The drawing under review shows one solid part. Ordinate dimensions are in mm from its lowest x, y, z. A direction names the side the tool comes from. Give positions to 0.01 mm unless a question says otherwise; leave off trailing zeros. Write each loop counter-clockwise with the first axis right and the second up, starting at its lowest first coordinate (ties: lowest second). Pieces come first, ordered by that corner, then holes. Notation, with made-up numbers: (58, -16) -> (86, -16) arc R26 ccw to (86, 14) -> close; hole circle Ø9 at (3.5, -20.5). An arc over 180 degrees is marked (long way). Write item = value, one per line.
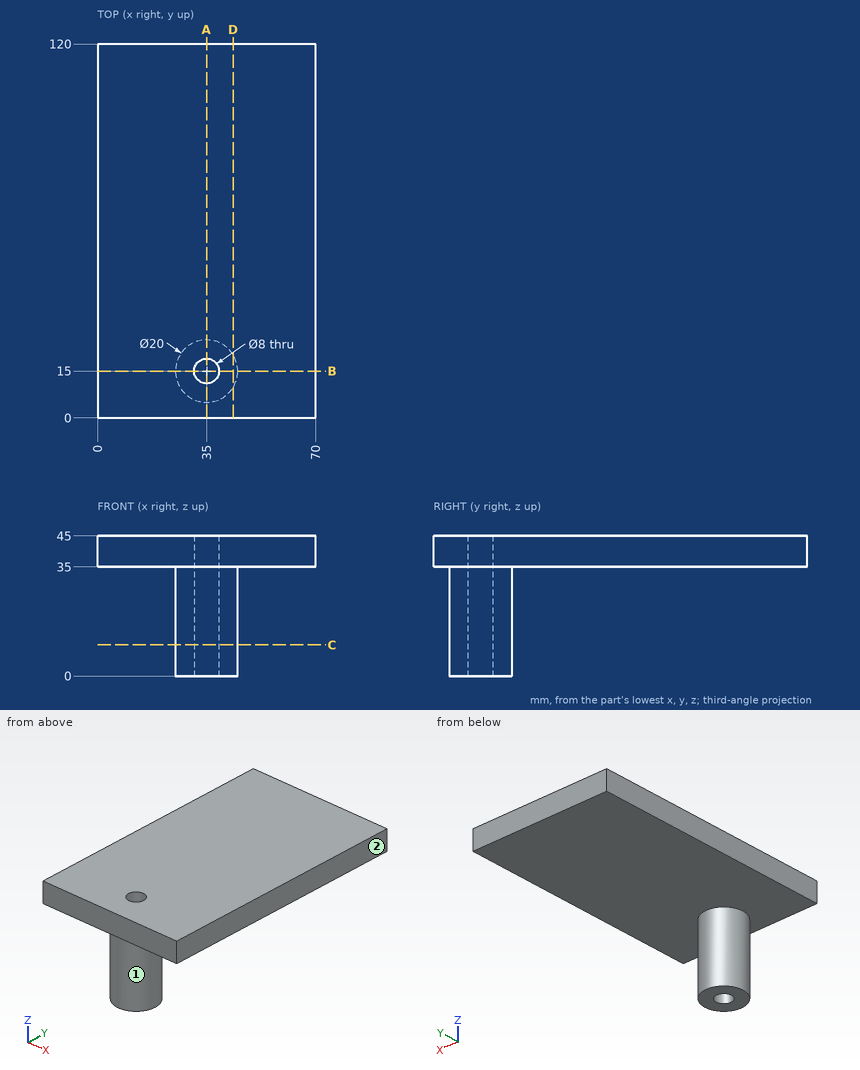
(1) To check wall thickness, follow probe 1 along Y at (x, z) = (35, 31); probe 2 along X at (y, z) = (15, 36); probe 3 along Z at (x, y) = (41, 61.5). State the ranges of each line that lie inside material, in increasing order.
Answers below:
probe_1 = 5 to 11, 19 to 25
probe_2 = 0 to 31, 39 to 70
probe_3 = 35 to 45
(2) Take a section at C-C (z = 10). Write out the cut boundary in (x, y), plus the area to 3 significant figures.
Answers below:
outline = circle Ø20 at (35, 15); hole circle Ø8 at (35, 15)
area = 264 mm^2
(3) Tool access review of the marked faces 1 and 2: name each direction out of +Z, -Z, +X, -X, +Y, -Y from which nothing blocks a thin tool from reaching the whole face with its end or side.
Answers below:
face_1 = -Z
face_2 = +Z, -Z, +X, +Y, -Y
(4) Take a section at D-D (x = 43.5). Write out the cut boundary in (y, z), plus the area to 3 significant figures.
Answers below:
outline = (0, 35) -> (9.73, 35) -> (9.73, 0) -> (20.27, 0) -> (20.27, 35) -> (120, 35) -> (120, 45) -> (0, 45) -> close
area = 1,570 mm^2
(5) For pin 1 (8 mm diameter, centred on x = 13.5, z = 27.5, fed in from +Y); pin 2 (3 mm diameter, centred on x = 15.5, y = 34.5, fed in from -Z), all flat-tipped, find the tip position at first contact; note any pin that passes through.
Answers below:
pin_1 = through
pin_2 = 35
(6) Take a section at B-B (y = 15). Write out the cut boundary in (x, z), plus the area to 3 significant figures.
Answers below:
outline = (0, 35) -> (25, 35) -> (25, 0) -> (31, 0) -> (31, 45) -> (0, 45) -> close; (39, 0) -> (45, 0) -> (45, 35) -> (70, 35) -> (70, 45) -> (39, 45) -> close
area = 1,040 mm^2
(7) Take a section at A-A (x = 35). Write out the cut boundary in (y, z), plus the area to 3 significant figures.
Answers below:
outline = (0, 35) -> (5, 35) -> (5, 0) -> (11, 0) -> (11, 45) -> (0, 45) -> close; (19, 0) -> (25, 0) -> (25, 35) -> (120, 35) -> (120, 45) -> (19, 45) -> close
area = 1,540 mm^2
